```python
from build123d import *

# Parameters (mm, degrees)
BOSS_EXTRUDE1_DEPTH      = 70
CUT_EXTRUDE2_DEPTH       = 211.416254125
CUT_EXTRUDE2_DEPTH_BACK  = 211.416254125
SKETCH2_W                = 100.4
SKETCH2_H                = 20.4
CUT_EXTRUDE3_DEPTH       = 20
FILLET1_R                = 45
CUT_EXTRUDE4_DEPTH       = 211.416254125
CUT_EXTRUDE4_DEPTH_BACK  = 211.416254125
BOSS_EXTRUDE2_DEPTH      = 70
SKETCH33_R               = 2.3
CUT_EXTRUDE9_DEPTH       = 10
SKETCH34_R               = 2.3
CUT_EXTRUDE10_DEPTH      = 10
FILLET2_R                = 5
CUT_EXTRUDE6_DEPTH       = 5
FILLET3_START            = 72
FILLET3_DEPTH            = 42
FILLET3_START_2          = 73.456949031
FILLET3_2_DEPTH          = 10
FILLET3_START_3          = 108.456949031
FILLET3_3_DEPTH          = 5
SKETCH31_R               = 2.3
CUT_EXTRUDE7_DEPTH       = 10
SKETCH32_R               = 2.3
CUT_EXTRUDE8_DEPTH       = 10
SKETCH35_R               = 2.3
CUT_EXTRUDE11_DEPTH      = 163.520229183
SKETCH36_R               = 4
CUT_EXTRUDE12_DEPTH      = 167.02180224
CUT_EXTRUDE13_DEPTH      = 211.416254158
CUT_EXTRUDE13_DEPTH_BACK = 211.416254158
SKETCH37_R               = 1.7
SKETCH38_R               = 2.3
CUT_EXTRUDE14_DEPTH      = 205.633819321
SKETCH39_R               = 4
CUT_EXTRUDE15_DEPTH      = 46
SKETCH40_R               = 3
CUT_EXTRUDE16_DEPTH      = 210.119583046


with BuildPart() as part:
    # Sketch1 → Boss-Extrude1 (new body)
    with BuildSketch(Plane(origin=(0, 0, 0), x_dir=(1, 0, 0), z_dir=(0, 1, 0))):
        Polygon((0, 0), (150, 0), (75, 129.903810568), align=None)
    extrude(amount=-BOSS_EXTRUDE1_DEPTH)

    # Sketch4 → Cut-Extrude2 (cut, two sides: drawn at the far end of the back side and taken through both)
    with BuildSketch(Plane(origin=(0, 0, 0), x_dir=(1, 0, 0), z_dir=(0, 1, 0)).offset(-CUT_EXTRUDE2_DEPTH_BACK)):
        Polygon((58.511973189, 45.566570047), (40.845863577, 35.365169595), (51.047264029, 17.699059984), (68.713373641, 27.900460435), align=None)
    extrude(amount=CUT_EXTRUDE2_DEPTH + CUT_EXTRUDE2_DEPTH_BACK, mode=Mode.SUBTRACT)

    # Sketch2 → Cut-Extrude3 (cut)
    with BuildSketch(Plane(origin=(0, 0, 0), x_dir=(1, 0, 0), z_dir=(0, 1, 0))):
        Polygon((109.197045256, 138.33483042), (58.997045256, 51.38587988), (41.330127019, 61.58587988), (91.530127019, 148.53483042), align=None)
        with Locations((124.2, 15.2)):
            Rectangle(SKETCH2_W, SKETCH2_H)
    extrude(amount=-CUT_EXTRUDE3_DEPTH, mode=Mode.SUBTRACT)

    # Fillet1
    fillet1_edges = [part.edges().sort_by_distance(p)[0] for p in [
        (0, -35, 0),
    ]]
    fillet(fillet1_edges, radius=FILLET1_R)

    # Sketch27 → Cut-Extrude4 (cut, two sides: drawn at the far end of the back side and taken through both)
    with BuildSketch(Plane(origin=(0, 0, 0), x_dir=(1, 0, 0), z_dir=(0, 1, 0)).offset(-CUT_EXTRUDE4_DEPTH_BACK)):
        Polygon((238.272822489, 351.900634614), (92.551448183, 99.503810568), (65.734741667, 53.05591239), (78.81753352, 30.4), (132.448551817, 30.4), (423.891300428, 30.4), (928.68494852, 321.842748611), (743.066470581, 643.343383225), align=None)
    extrude(amount=CUT_EXTRUDE4_DEPTH + CUT_EXTRUDE4_DEPTH_BACK, mode=Mode.SUBTRACT)

    # Sketch28 → Boss-Extrude2 (add)
    with BuildSketch(Plane(origin=(0, 0, 0), x_dir=(1, 0, 0), z_dir=(0, 1, 0))):
        Polygon((83.054457118, 83.054539524), (113.460135283, 30.4), (107.686368323, 30.4), (80.167837876, 78.054768335), align=None)
    extrude(amount=-BOSS_EXTRUDE2_DEPTH)

    # Sketch33 → Cut-Extrude9 (cut)
    with BuildSketch(Plane(origin=(26.327172275, 0, 15.2), x_dir=(0.4999999999999997, 0, -0.8660254037844388), z_dir=(0.8660254037844389, 0, 0.49999999999999983))):
        with Locations((122.448551817, -10)):
            Circle(SKETCH33_R)
    extrude(amount=-CUT_EXTRUDE9_DEPTH, mode=Mode.SUBTRACT)

    # Sketch34 → Cut-Extrude10 (cut)
    with BuildSketch(Plane(origin=(0, 0, -30.4), x_dir=(-1, 0, 0), z_dir=(0, 0, -1))):
        with Locations((-122.448551817, -10)):
            Circle(SKETCH34_R)
    extrude(amount=-CUT_EXTRUDE10_DEPTH, mode=Mode.SUBTRACT)

    # Fillet2
    fillet2_edges = [part.edges().sort_by_distance(p)[0] for p in [
        (83.054457118, -35, -83.054539524),
        (80.167837876, -35, -78.054768335),
        (65.734741667, -35, -53.05591239),
        (78.81753352, -35, -30.4),
        (107.686368323, -35, -30.4),
        (113.460135283, -35, -30.4),
    ]]
    fillet(fillet2_edges, radius=FILLET2_R)

    # Sketch30 → Cut-Extrude6 (cut)
    with BuildSketch(Plane.XZ.offset(70)):
        Polygon((62.116998953, -39.323625207), (122.736002524, -74.32843068), (125.736414421, -69.132516088), (65.117410851, -34.127710616), align=None)
    extrude(amount=-CUT_EXTRUDE6_DEPTH, mode=Mode.SUBTRACT)

    # Fillet3: read off the stored shape, not the designer's step
    # Fillet3 outline → Fillet3 (cut)
    with BuildSketch(Plane(origin=(0, 0, 0), x_dir=(0.5000686496051991, 0, 0.8659857652883406), z_dir=(0.8659857652883404, 0, -0.5000686496051993)).offset(FILLET3_START)):
        with BuildLine():
            Line((-2.990935885, 70), (-5.490935885, 70))
            ThreePointArc((-5.490935885, 70), (-3.723168932, 69.267766953), (-2.990935885, 67.5))
            Line((-2.990935885, 67.5), (-2.990935885, 70))
        make_face()
        with BuildLine():
            Line((5.509064115, 70), (3.009064115, 70))
            Line((3.009064115, 70), (3.009064115, 67.5))
            ThreePointArc((3.009064115, 67.5), (3.741297162, 69.267766953), (5.509064115, 70))
        make_face()
    extrude(amount=FILLET3_DEPTH, mode=Mode.SUBTRACT)

    # Fillet3 2 outline → Fillet3 2 (add)
    with BuildSketch(Plane(origin=(0, 0, 0), x_dir=(0.5000686496051991, 0, 0.8659857652883406), z_dir=(0.8659857652883404, 0, -0.5000686496051993)).offset(FILLET3_START_2)):
        with BuildLine():
            ThreePointArc((-0.490935885, 65), (-2.258702838, 65.732233047), (-2.990935885, 67.5))
            Line((-2.990935885, 67.5), (-2.990935885, 65))
            Line((-2.990935885, 65), (-0.490935885, 65))
        make_face()
        with BuildLine():
            ThreePointArc((3.009064115, 67.5), (2.276831068, 65.732233047), (0.509064115, 65))
            Line((0.509064115, 65), (3.009064115, 65))
            Line((3.009064115, 65), (3.009064115, 67.5))
        make_face()
    extrude(amount=FILLET3_2_DEPTH)

    # Fillet3 3 outline → Fillet3 3 (add)
    with BuildSketch(Plane(origin=(0, 0, 0), x_dir=(0.5000686496051991, 0, 0.8659857652883406), z_dir=(0.8659857652883404, 0, -0.5000686496051993)).offset(FILLET3_START_3)):
        with BuildLine():
            ThreePointArc((-0.490935885, 65), (-2.258702838, 65.732233047), (-2.990935885, 67.5))
            Line((-2.990935885, 67.5), (-2.990935885, 65))
            Line((-2.990935885, 65), (-0.490935885, 65))
        make_face()
        with BuildLine():
            ThreePointArc((3.009064115, 67.5), (2.276831068, 65.732233047), (0.509064115, 65))
            Line((0.509064115, 65), (3.009064115, 65))
            Line((3.009064115, 65), (3.009064115, 67.5))
        make_face()
    extrude(amount=FILLET3_3_DEPTH)

    # Sketch31 → Cut-Extrude7 (cut)
    with BuildSketch(Plane(origin=(4.330127019, 0, 2.5), x_dir=(0.5000000000000019, 0, -0.8660254037844376), z_dir=(0.8660254037844376, 0, 0.5000000000000019))):
        with Locations((89, -10)):
            Circle(SKETCH31_R)
        with Locations((132.113248654, -10)):
            Circle(SKETCH31_R)
    extrude(amount=-CUT_EXTRUDE7_DEPTH, mode=Mode.SUBTRACT)

    # Sketch32 → Cut-Extrude8 (cut)
    with BuildSketch(Plane(origin=(0, 0, -5), x_dir=(-1, 0, 0), z_dir=(0, 0, -1))):
        with Locations((-132.113248654, -10)):
            Circle(SKETCH32_R)
        with Locations((-89, -10)):
            Circle(SKETCH32_R)
    extrude(amount=-CUT_EXTRUDE8_DEPTH, mode=Mode.SUBTRACT)

    # Sketch35 → Cut-Extrude11 (cut, through all)
    with BuildSketch(Plane(origin=(45.946562611, 0, -26.532116854), x_dir=(-0.5000686496051995, 0, -0.8659857652883403), z_dir=(0.8659857652883401, 0, -0.5000686496051994))):
        with Locations((0, -15)):
            Circle(SKETCH35_R)
        with Locations((0, -55)):
            Circle(SKETCH35_R)
    extrude(amount=-CUT_EXTRUDE11_DEPTH, mode=Mode.SUBTRACT)

    # Sketch36 → Cut-Extrude12 (cut, through all)
    with BuildSketch(Plane(origin=(42.482619549, 0, -24.531842256), x_dir=(-0.5000686496051995, 0, -0.8659857652883403), z_dir=(0.8659857652883401, 0, -0.5000686496051994))):
        with Locations((0, -15)):
            Circle(SKETCH36_R)
        with Locations((0, -55)):
            Circle(SKETCH36_R)
    extrude(amount=-CUT_EXTRUDE12_DEPTH, mode=Mode.SUBTRACT)

    # Sketch37 → Cut-Extrude13 (cut, two sides: drawn at the far end of the back side and taken through both)
    with BuildSketch(Plane.XZ.offset(70).offset(-CUT_EXTRUDE13_DEPTH_BACK)):
        with Locations(Location((69.166562249, -15.2, 0), (0, 0, 270))):
            Circle(SKETCH37_R)
        with Locations(Location((105.195419079, -15.2, 0), (0, 0, 270))):
            Circle(SKETCH37_R)
        with Locations(Location((47.746867262, -52.3, 0), (0, 0, 270))):
            Circle(SKETCH37_R)
        with Locations(Location((65.761295677, -83.501905284, 0), (0, 0, 270))):
            Circle(SKETCH37_R)
    extrude(amount=CUT_EXTRUDE13_DEPTH + CUT_EXTRUDE13_DEPTH_BACK, mode=Mode.SUBTRACT)

    # Sketch38 → Cut-Extrude14 (cut, through all)
    with BuildSketch(Plane(origin=(0, -20, 0), x_dir=(1, 0, 0), z_dir=(0, 1, 0))):
        with Locations(Location((89, 15.2, 0), (0, 0, 270))):
            Circle(SKETCH38_R)
        with Locations(Location((126.224275908, 15.2, 0), (0, 0, 270))):
            Circle(SKETCH38_R)
        with Locations(Location((76.275724092, 101.713429511, 0), (0, 0, 270))):
            Circle(SKETCH38_R)
        with Locations(Location((57.663586138, 69.476260937, 0), (0, 0, 270))):
            Circle(SKETCH38_R)
    extrude(amount=-CUT_EXTRUDE14_DEPTH, mode=Mode.SUBTRACT)

    # Sketch39 → Cut-Extrude15 (cut)
    with BuildSketch(Plane.XZ.offset(70)):
        with Locations(Location((89, -15.2, 0), (0, 0, 270))):
            Circle(SKETCH39_R)
        with Locations(Location((126.224275908, -15.2, 0), (0, 0, 270))):
            Circle(SKETCH39_R)
        with Locations(Location((57.663586138, -69.476260937, 0), (0, 0, 270))):
            Circle(SKETCH39_R)
        with Locations(Location((76.275724092, -101.713429511, 0), (0, 0, 270))):
            Circle(SKETCH39_R)
    extrude(amount=-CUT_EXTRUDE15_DEPTH, mode=Mode.SUBTRACT)

    # Sketch40 → Cut-Extrude16 (cut, through all)
    with BuildSketch(Plane(origin=(0, -66, 0), x_dir=(-1, 0, 0), z_dir=(0, -1, 0))):
        with Locations(Location((-65.761295677, 83.501905284, 0), (0, 0, 90))):
            Circle(SKETCH40_R)
        with Locations(Location((-47.746867262, 52.3, 0), (0, 0, 90))):
            Circle(SKETCH40_R)
        with Locations(Location((-69.166562249, 15.2, 0), (0, 0, 90))):
            Circle(SKETCH40_R)
        with Locations(Location((-105.195419079, 15.2, 0), (0, 0, 90))):
            Circle(SKETCH40_R)
    extrude(amount=-CUT_EXTRUDE16_DEPTH, mode=Mode.SUBTRACT)


solid = part.part
```
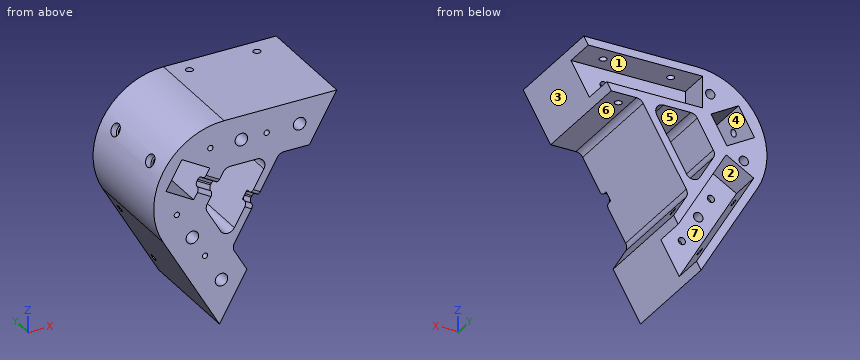
Geometry: final body of the model. Coordinates: model frame, mm. Face numbers are marked on the shaded views. A direction names the side the tool comes from. Round coordinates to 2 decimals unless told otherwise and drop trailing zeros. Write each loop counter-clockwise with the first axis right and the second up, starting at its lowest first coordinate (ties: lowest second). Pieces come first, ordered by that corner, then holes. Notation, with made-up numbers: (66.5, -5) -> (80.5, -5) arc R10 ccw to (80.5, 14) -> close; hole circle Ø3 at (-12, -31.75). An arc over 180 degrees is marked (long way). Use CSV: the item, a comma, the result in double quotes. Start each with the question number.
Q1. Pull-direction query (X, two-part tool) for the marked faces 1, 2, 3 and 4; classes: pulls with the +X half, pulls with the -X half, needs draft (parallel to the pull), parting line crosses it, or undercut.
Q2. Section A-A (x = 118). Return loops of the section in (y, z).
Q3. Line query: L1, parallel to Z at x = 54, y = -55.5; L2, parallel to X at y = -53, z = -72; L3, parallel to X at y = -21.5, z = -54. Output: solid intervals per line, ascending.
Q4. Reachability of the marked faces 5, 6 and 7 from +Z, -Z, +X, -X, +Y, -Y: full face, straight path, thin tool, end or side. Return the list, or none.
Q5. Section C-C (y = -32.5). Give the number of separate pieces and of enclosed holes in the cut face, plus the area to 3 significant figures.
Q6. Section B-B (z = -63.5). Return loops of the section in (x, y), plus the area to 3 significant figures.
Q7. First-contact query: pin 1 Ø6.5 at (x, z) = (104.5, -14) entering from +Y; pin 2 Ø8 at (y, z) = (-25, -96.5) entering from -X; pin 3 Ø4 at (x, z) = (77, -101) entering from -Y. Flat tips, straight axial feed; report the tip coordinate or a pass-through.
Result sheet:
1,face 1,"needs draft"
1,face 2,"undercut"
1,face 3,"pulls with the +X half"
1,face 4,"undercut"
2,outline,"(-70, -30.4) -> (0, -30.4) -> (0, -25.4) -> (-20, -25.4) -> (-20, -5) -> (0, -5) -> (0, 0) -> (-70, 0) -> close"
3,L1,"-93.53 to -71.08, -67.87 to -42.96, -19.4 to -6.9"
3,L2,"41.57 to 54.56, 60.77 to 77.1, 83.24 to 89.44"
3,L3,"33.85 to 45.28, 50.22 to 66.6, 94.06 to 99.83"
4,face 5,"+Y, -Y"
4,face 6,"-Z, +X, +Y, -Y"
4,face 7,"+Y"
5,separate pieces,"1"
5,enclosed holes,"10"
5,area,"5,490 mm²"
6,outline,"(36.92, -70) -> (71.76, -70) -> (71.76, 0) -> (65.99, 0) -> (65.99, -20) -> (42.44, -20) -> (42.44, 0) -> (36.92, 0) -> close; (88.57, -70) -> (94.35, -70) -> (94.35, 0) -> (88.57, 0) -> close"
6,area,"2,370 mm²"
7,pin 1,"y = -20"
7,pin 2,"x = 53.4"
7,pin 3,"y = -24"
